Autodesk Inventor part; units mm, degrees
ref_plane "YZ Plane" through (0, 0, 0) normal (1, 0, 0) x (0, 1, 0)
ref_plane "XZ Plane" through (0, 0, 0) normal (0, 1, 0) x (-1, 0, 0)
ref_plane "XY Plane" through (0, 0, 0) normal (0, 0, 1) x (1, 0, 0)
sketch "Sketch2" plane through (0, 0, 0) normal (0, 1, 0) x (-1, 0, 0)
  line L0 (0, 0) -> (-114.3, 0)
  line L1 (-114.3, 0) -> (-114.3, -152.4)
  line L2 (-114.3, -152.4) -> (0, -152.4)
  line L3 (0, -152.4) -> (0, 0)
  dimension "d1" = 152.4
  dimension "d2" = 114.3
extrude "Extrusion1" add sketch "Sketch2" against normal blind 19.05
sketch "Sketch3" plane through (0, 0, 0) normal (0, 1, 0) x (1, 0, 0)
  line L0 (114.3, 0) -> (114.3, 152.4)
  line L1 (114.3, 152.4) -> (0, 152.4)
  line L2 (0, 0) -> (114.3, 0)
  line L3 (114.3, 152.4) -> (114.3, 0)
  line L4 (0, 152.4) -> (114.3, 152.4)
  line L5 (114.3, 0) -> (88.9, 0)
  line L6 (88.9, 0) -> (88.9, 152.4)
  line L7 (88.9, 152.4) -> (114.3, 152.4)
  line L8 (114.3, 152.4) -> (114.3, 0)
  point P0 (88.9, 0)
  dimension "d5" = 25.4
extrude "Extrusion2" add sketch "Sketch3" along normal blind 203.2
sketch "Sketch4" plane through (114.3, -19.05, 0) normal (1, 0, 0) x (0, 0, -1)
  line L0 (0, 222.25) -> (152.4, 222.25) construction
  line L1 (76.2, 222.25) -> (76.2, 0) construction
  line L2 (152.4, 0) -> (0, 0) construction
  point P0 (0, 19.05)
  point P1 (76.2, 196.85)
  dimension "d8" = 25.4
hole "Hole1" at (114.3, 177.8, -76.2) direction (-1, 0, 0) diameter 19.8374 end through all
properties part number "oneHalfForkSupport" material "Wood (Birch)"
The model under review builds one solid part; all positions refer to its coordinate system, in mm. A direction names the side the tool comes from. Give positions to 0.01 mm unless a question says otherwise; leave off trailing zeros. Write each loop counter-clockwise with the first axis right and the second up, starting at its lowest first coordinate (ties: lowest second). Pieces come first, ordered by that corner, then holes. Notation, with made-up numbers: M -5,-19.75 L 20,-19.75 A36 cw 20,17.25 Z; hole C 9.5,20.25 d5. An arc over 180 degrees is marked long. Write each question's results on one line, items separated by ' | '. Start each with the question number.
1. For faces 1 (the flat face through (88.9, 100, -75)), 2 (the flat face through (91, 68, -152.4)), list the 3-axis set-ups (+Z, -Z, +X, -X, +Y, -Y) from which the entire face can be reached by the end or side of a thin tool; tool diameter is ignored.
2. For probe 1 along Z at (x, y) = (99, 177); probe 2 along Y at (x, z) = (95, -76); probe 3 along X at (y, z) = (185, -34), list the stretches that pass through material, from the lowest coordinate up. Write a range as [from, to].
3. We need section C-C (y = 74). Write out the cut boundary in (x, z).
4. Insertion check: pin 1 Ø10 at (x, z) = (26.5, -112.5) entering from +Y; pin 2 Ø12 at (y, z) = (177.8, -76.2) entering from +X. Each pin has a flat end and moves straight along its axis. Give the tip position at first contact, or say it passes through.
5. We need section A-A (z = -76.2). Write out the cut boundary in (x, y).
6. Mouldability with a two-part tool opening along Y and no side actions: class faces 3 (the flat face through (114.3, 94, -75)), 4 (the cylindrical face through (101.42, 174.82, -85.66)), 5 (the flat face through (58, -19.05, -75)), 6 (the flat face through (45, 0, -75)) as released by +Y, released by -Y, zero draft, split by the parting line, or undercut.
7. We need section B-B (y = 177.8). Write out the cut boundary in (x, z).
8. We need section D-D (z = -54). Write out the cut boundary in (x, y), and give its area (3 significant figures).
Results found:
1) face 1: +Z, -Z, -X, +Y | face 2: -Z, +X, -X, +Y, -Y
2) probe 1: z = [-152.4, -86.09], [-66.31, 0] | probe 2: y = [-19.05, 167.88], [187.72, 203.2] | probe 3: x = [88.9, 114.3]
3) outline: M 88.9,-152.4 L 114.3,-152.4 L 114.3,0 L 88.9,0 Z
4) pin 1: stops at y = 0 | pin 2: passes through
5) outline: M 0,-19.05 L 114.3,-19.05 L 114.3,167.88 L 88.9,167.88 L 88.9,0 L 0,0 Z; M 88.9,187.72 L 114.3,187.72 L 114.3,203.2 L 88.9,203.2 Z
6) face 3: zero draft | face 4: undercut | face 5: released by -Y | face 6: released by +Y
7) outline: M 88.9,-152.4 L 114.3,-152.4 L 114.3,-86.12 L 88.9,-86.12 Z; M 88.9,-66.28 L 114.3,-66.28 L 114.3,0 L 88.9,0 Z
8) outline: M 0,-19.05 L 114.3,-19.05 L 114.3,203.2 L 88.9,203.2 L 88.9,0 L 0,0 Z | area: 7,340 mm^2
